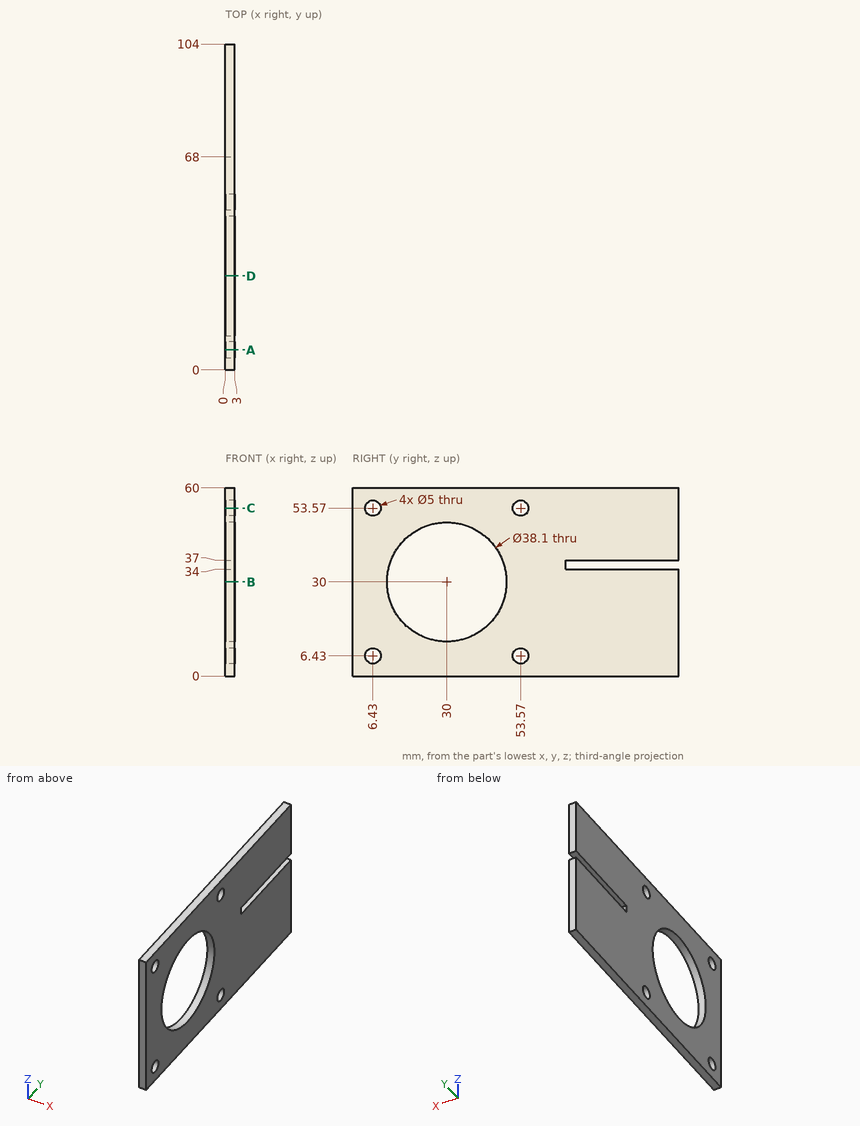
Check sheet for the drawn part. Datum: minimum x, y, z corner. Units: mm. Round coordinates to 2 decimals unless told otherwise and drop trailing zeros. Order: outer loops, then holes, each group sorted by start corner. A loop starts at its lowest first (then second) coordinate and runs counter-clockwise, first axis right, second up.
1) Scan lines: line 1 (Y direction, x = 1.7, z = 6.5); line 2 (Z direction, x = 2.3, y = 6.43); line 3 (Z direction, x = 1.5, y = 77.5). Record each from-to range of solid material in increasing order.
2) Section check C-C (z = 53.57). Record the boundary of the cut face in (x, y), and give its area (3 significant figures).
3) Section check B-B (z = 30). Record the boundary of the cut face in (x, y).
4) Section check D-D (y = 30). Record the boundary of the cut face in (x, z), and give its area (3 significant figures).
5) Go/stop test with a flat-tipped pin: pin 1 Ø1.5 at (x, z) = (1, 35.5) entering from +Y. Record where the tip stops, or that it passes through.
6) Section check A-A (y = 6.43). Record the boundary of the cut face in (x, z).
Result:
1. line 1: y = 0 to 3.93, 8.93 to 51.07, 56.07 to 104
1. line 2: z = 0 to 3.93, 8.93 to 51.07, 56.07 to 60
1. line 3: z = 0 to 34, 37 to 60
2. outline: (0, 0) - (3, 0) - (3, 3.93) - (0, 3.93) - close; (0, 8.93) - (3, 8.93) - (3, 51.07) - (0, 51.07) - close; (0, 56.07) - (3, 56.07) - (3, 104) - (0, 104) - close
2. area: 282 mm2
3. outline: (0, 0) - (3, 0) - (3, 10.95) - (0, 10.95) - close; (0, 49.05) - (3, 49.05) - (3, 104) - (0, 104) - close
4. outline: (0, 0) - (3, 0) - (3, 10.95) - (0, 10.95) - close; (0, 49.05) - (3, 49.05) - (3, 60) - (0, 60) - close
4. area: 65.7 mm2
5. pin 1: stops at y = 68
6. outline: (0, 0) - (3, 0) - (3, 3.93) - (0, 3.93) - close; (0, 8.93) - (3, 8.93) - (3, 51.07) - (0, 51.07) - close; (0, 56.07) - (3, 56.07) - (3, 60) - (0, 60) - close
